The listing builds one solid part. Answer for the finished solid, in the listing's coordinates (mm). Face numbers are marked on the shaded views. Give positions to 0.01 mm unless a question says otherwise; leave off trailing zeros. Put each result on its own line as item: value. Start each with the question number.
1) A cutting plane is placed at A-A (y = 2.5). Give the number of separate pieces and of enclosed holes in the cut face, then the cut area to 3 significant figures.
2) For a pull along Z with two mould halves and no side action, classify the marked faces 1 and 2 as released by +Z, released by -Z, zero draft, split by the parting line, or undercut.
3) Find the intervals of material crossed by line 1 along Z through (x, y) = (6, 2); line 2 along X through (y, z) = (4, 35); line 3 along Z through (x, y) = (-2.5, 3), in increasing order. Write a range as from..to.
4) Flat-ended cylindrical pins translate along their axes: pin 1 Ø2.5 at (y, z) = (2, -35) entering from +X; pin 2 Ø4 at (x, z) = (5.13, 14.1) entering from +Y; pin 3 Ø1 at (y, z) = (3, 9.5) entering from -X. Find the tip coordinate at first contact, or state that the pin passes through.
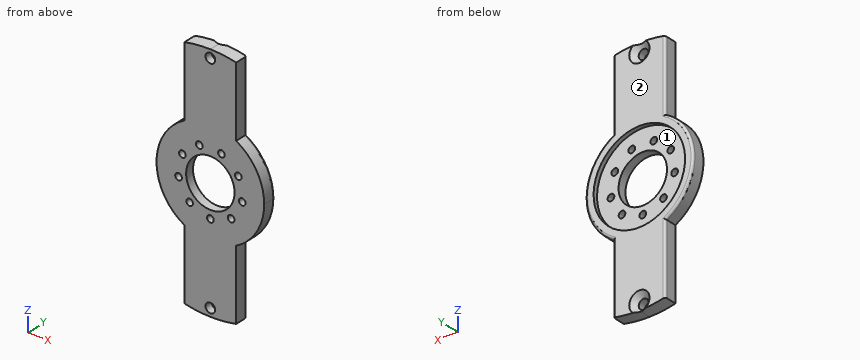
from build123d import *

# Parameters (mm, degrees)
BOSS_EXTRUDE2_DEPTH                             = 6
CSK_FOR_M4_FLAT_HEAD_MACHINE_SCREW1_D           = 4.5
CSK_FOR_M4_FLAT_HEAD_MACHINE_SCREW1_CSINK_D     = 9.4
CSK_FOR_M4_FLAT_HEAD_MACHINE_SCREW1_CSINK_ANGLE = 90
SKETCH7_R                                       = 21.25
CUT_EXTRUDE2_DEPTH                              = 2
SKETCH8_R                                       = 11.25
CUT_EXTRUDE3_DEPTH                              = 62.457302349
SKETCH9_R                                       = 1.55
CUT_EXTRUDE4_DEPTH                              = 62.457302349
FILLET1_R                                       = 1


with BuildPart() as part:
    # Sketch2 → Boss-Extrude2 (new body)
    with BuildSketch(Plane(origin=(0, 0, 0), x_dir=(1, 0, 0), z_dir=(0, 1, 0))):
        with BuildLine():
            ThreePointArc((0, -50), (-6.044327096, -49.633316532), (-12, -48.538644398))
            Line((-12, -48.538644398), (-12, -54.699177325))
            ThreePointArc((-12, -54.699177325), (-6.035149949, -55.673844533), (0, -56))
            Line((0, -56), (0, -54.269322199))
            ThreePointArc((0, -54.269322199), (-2, -52.269322199), (0, -50.269322199))
            Line((0, -50.269322199), (0, -50))
        make_face()
        with BuildLine():
            ThreePointArc((2, -52.269322199), (1.414213562, -50.855108637), (0, -50.269322199))
            Line((0, -50.269322199), (0, -54.269322199))
            ThreePointArc((0, -54.269322199), (1.414213562, -53.683535761), (2, -52.269322199))
        make_face()
        with BuildLine():
            Line((0, -54.269322199), (0, -50.269322199))
            ThreePointArc((0, -50.269322199), (-2, -52.269322199), (0, -54.269322199))
        make_face()
        with BuildLine():
            ThreePointArc((2, -52.269322199), (1.414213562, -50.855108637), (0, -50.269322199))
            Line((0, -50.269322199), (0, -54.269322199))
            ThreePointArc((0, -54.269322199), (1.414213562, -53.683535761), (2, -52.269322199))
        make_face()
        with BuildLine():
            Line((0, -54.269322199), (0, -50.269322199))
            ThreePointArc((0, -50.269322199), (-2, -52.269322199), (0, -54.269322199))
        make_face()
        with BuildLine():
            Line((12, -54.699177325), (12, -48.538644398))
            ThreePointArc((12, -48.538644398), (6.044327096, -49.633316532), (0, -50))
            Line((0, -50), (0, -50.269322199))
            ThreePointArc((0, -50.269322199), (1.414213562, -50.855108637), (2, -52.269322199))
            ThreePointArc((2, -52.269322199), (1.414213562, -53.683535761), (0, -54.269322199))
            Line((0, -54.269322199), (0, -56))
            ThreePointArc((0, -56), (6.035149949, -55.673844533), (12, -54.699177325))
        make_face()
        with BuildLine():
            Line((0, -48.538644398), (-12, -48.538644398))
            ThreePointArc((-12, -48.538644398), (-6.044327096, -49.633316532), (0, -50))
            Line((0, -50), (0, -48.538644398))
        make_face()
        with BuildLine():
            Line((12, -48.538644398), (0, -48.538644398))
            Line((0, -48.538644398), (0, -50))
            ThreePointArc((0, -50), (6.044327096, -49.633316532), (12, -48.538644398))
        make_face()
        with BuildLine():
            ThreePointArc((0, -25), (-6.193028137, -24.220784514), (-12, -21.931712199))
            Line((-12, -21.931712199), (-12, -48.538644398))
            Line((-12, -48.538644398), (0, -48.538644398))
            Line((0, -48.538644398), (0, -25))
        make_face()
        with BuildLine():
            ThreePointArc((12, -21.931712199), (6.193028137, -24.220784514), (0, -25))
            Line((0, -25), (0, -48.538644398))
            Line((0, -48.538644398), (12, -48.538644398))
            Line((12, -48.538644398), (12, -21.931712199))
        make_face()
        with BuildLine():
            Line((0, -48.538644398), (-12, -48.538644398))
            ThreePointArc((-12, -48.538644398), (-6.044327096, -49.633316532), (0, -50))
            Line((0, -50), (0, -48.538644398))
        make_face()
        with BuildLine():
            Line((12, -48.538644398), (0, -48.538644398))
            Line((0, -48.538644398), (0, -50))
            ThreePointArc((0, -50), (6.044327096, -49.633316532), (12, -48.538644398))
        make_face()
        with BuildLine():
            ThreePointArc((-12, 48.538644398), (-6.044327096, 49.633316532), (0, 50))
            Line((0, 50), (0, 50.269322199))
            ThreePointArc((0, 50.269322199), (-2, 52.269322199), (0, 54.269322199))
            Line((0, 54.269322199), (0, 56))
            ThreePointArc((0, 56), (-6.035149949, 55.673844533), (-12, 54.699177325))
            Line((-12, 54.699177325), (-12, 48.538644398))
        make_face()
        with BuildLine():
            ThreePointArc((0, 54.269322199), (-2, 52.269322199), (0, 50.269322199))
            Line((0, 50.269322199), (0, 54.269322199))
        make_face()
        with BuildLine():
            Line((0, 54.269322199), (0, 50.269322199))
            ThreePointArc((0, 50.269322199), (1.414213562, 50.855108637), (2, 52.269322199))
            ThreePointArc((2, 52.269322199), (1.414213562, 53.683535761), (0, 54.269322199))
        make_face()
        with BuildLine():
            ThreePointArc((0, 54.269322199), (-2, 52.269322199), (0, 50.269322199))
            Line((0, 50.269322199), (0, 54.269322199))
        make_face()
        with BuildLine():
            Line((0, 54.269322199), (0, 50.269322199))
            ThreePointArc((0, 50.269322199), (1.414213562, 50.855108637), (2, 52.269322199))
            ThreePointArc((2, 52.269322199), (1.414213562, 53.683535761), (0, 54.269322199))
        make_face()
        with BuildLine():
            Line((0, 50.269322199), (0, 50))
            ThreePointArc((0, 50), (6.044327096, 49.633316532), (12, 48.538644398))
            Line((12, 48.538644398), (12, 54.699177325))
            ThreePointArc((12, 54.699177325), (6.035149949, 55.673844533), (0, 56))
            Line((0, 56), (0, 54.269322199))
            ThreePointArc((0, 54.269322199), (1.414213562, 53.683535761), (2, 52.269322199))
            ThreePointArc((2, 52.269322199), (1.414213562, 50.855108637), (0, 50.269322199))
        make_face()
        with BuildLine():
            Line((-12, 48.538644398), (0, 48.538644398))
            Line((0, 48.538644398), (0, 50))
            ThreePointArc((0, 50), (-6.044327096, 49.633316532), (-12, 48.538644398))
        make_face()
        with BuildLine():
            Line((0, 50), (0, 48.538644398))
            Line((0, 48.538644398), (12, 48.538644398))
            ThreePointArc((12, 48.538644398), (6.044327096, 49.633316532), (0, 50))
        make_face()
        with BuildLine():
            Line((-12, 48.538644398), (0, 48.538644398))
            Line((0, 48.538644398), (0, 50))
            ThreePointArc((0, 50), (-6.044327096, 49.633316532), (-12, 48.538644398))
        make_face()
        with BuildLine():
            Line((0, 50), (0, 48.538644398))
            Line((0, 48.538644398), (12, 48.538644398))
            ThreePointArc((12, 48.538644398), (6.044327096, 49.633316532), (0, 50))
        make_face()
        with BuildLine():
            Line((0, 25), (0, 48.538644398))
            Line((0, 48.538644398), (-12, 48.538644398))
            Line((-12, 48.538644398), (-12, 21.931712199))
            ThreePointArc((-12, 21.931712199), (-6.193028137, 24.220784514), (0, 25))
        make_face()
        with BuildLine():
            Line((12, 48.538644398), (0, 48.538644398))
            Line((0, 48.538644398), (0, 25))
            ThreePointArc((0, 25), (6.193028137, 24.220784514), (12, 21.931712199))
            Line((12, 21.931712199), (12, 48.538644398))
        make_face()
        with BuildLine():
            ThreePointArc((12, 21.931712199), (6.193028137, 24.220784514), (0, 25))
            Line((0, 25), (0, 21.25))
            ThreePointArc((0, 21.25), (15.0260191, 15.0260191), (21.25, 0))
            ThreePointArc((21.25, 0), (15.0260191, -15.0260191), (0, -21.25))
            Line((0, -21.25), (0, -25))
            ThreePointArc((0, -25), (6.193028137, -24.220784514), (12, -21.931712199))
            ThreePointArc((12, -21.931712199), (21.505813168, -12.747548784), (25, 0))
            ThreePointArc((25, 0), (21.505813168, 12.747548784), (12, 21.931712199))
        make_face()
        with BuildLine():
            Line((0, 21.25), (0, 25))
            ThreePointArc((0, 25), (-6.193028137, 24.220784514), (-12, 21.931712199))
            ThreePointArc((-12, 21.931712199), (-25, 0), (-12, -21.931712199))
            ThreePointArc((-12, -21.931712199), (-6.193028137, -24.220784514), (0, -25))
            Line((0, -25), (0, -21.25))
            ThreePointArc((0, -21.25), (-21.25, 0), (0, 21.25))
        make_face()
        with BuildLine():
            ThreePointArc((21.25, 0), (15.0260191, 15.0260191), (0, 21.25))
            Line((0, 21.25), (0, 0))
            Line((0, 0), (0, -21.25))
            ThreePointArc((0, -21.25), (15.0260191, -15.0260191), (21.25, 0))
        make_face()
        with BuildLine():
            Line((0, 0), (0, 21.25))
            ThreePointArc((0, 21.25), (-21.25, 0), (0, -21.25))
            Line((0, -21.25), (0, 0))
        make_face()
        with BuildLine():
            ThreePointArc((21.25, 0), (15.0260191, 15.0260191), (0, 21.25))
            Line((0, 21.25), (0, 0))
            Line((0, 0), (0, -21.25))
            ThreePointArc((0, -21.25), (15.0260191, -15.0260191), (21.25, 0))
        make_face()
        with BuildLine():
            Line((0, 0), (0, 21.25))
            ThreePointArc((0, 21.25), (-21.25, 0), (0, -21.25))
            Line((0, -21.25), (0, 0))
        make_face()
        with BuildLine():
            ThreePointArc((12, 21.931712199), (6.193028137, 24.220784514), (0, 25))
            Line((0, 25), (0, 21.25))
            ThreePointArc((0, 21.25), (15.0260191, 15.0260191), (21.25, 0))
            ThreePointArc((21.25, 0), (15.0260191, -15.0260191), (0, -21.25))
            Line((0, -21.25), (0, -25))
            ThreePointArc((0, -25), (6.193028137, -24.220784514), (12, -21.931712199))
            ThreePointArc((12, -21.931712199), (21.505813168, -12.747548784), (25, 0))
            ThreePointArc((25, 0), (21.505813168, 12.747548784), (12, 21.931712199))
        make_face()
        with BuildLine():
            Line((0, 21.25), (0, 25))
            ThreePointArc((0, 25), (-6.193028137, 24.220784514), (-12, 21.931712199))
            ThreePointArc((-12, 21.931712199), (-25, 0), (-12, -21.931712199))
            ThreePointArc((-12, -21.931712199), (-6.193028137, -24.220784514), (0, -25))
            Line((0, -25), (0, -21.25))
            ThreePointArc((0, -21.25), (-21.25, 0), (0, 21.25))
        make_face()
    extrude(amount=BOSS_EXTRUDE2_DEPTH)

    # CSK for M4 Flat Head Machine Screw1 (through all)
    with Locations(Plane(origin=(0, 6, 0), x_dir=(1, 0, 0), z_dir=(0, 1, 0))):
        with Locations((0, 52.269322197)):
            csk_for_m4_flat_head_machine_screw1 = CounterSinkHole(CSK_FOR_M4_FLAT_HEAD_MACHINE_SCREW1_D / 2, CSK_FOR_M4_FLAT_HEAD_MACHINE_SCREW1_CSINK_D / 2, counter_sink_angle=CSK_FOR_M4_FLAT_HEAD_MACHINE_SCREW1_CSINK_ANGLE)

    # Mirror1: CSK for M4 Flat Head Machine Screw1 across plane
    add(csk_for_m4_flat_head_machine_screw1.mirror(Plane.XY), mode=Mode.SUBTRACT)

    # Sketch7 → Cut-Extrude2 (cut)
    with BuildSketch(Plane(origin=(0, 6, 0), x_dir=(1, 0, 0), z_dir=(0, 1, 0))):
        with Locations(Location((0, 0, 0), (0, 0, 270))):
            Circle(SKETCH7_R)
    extrude(amount=-CUT_EXTRUDE2_DEPTH, mode=Mode.SUBTRACT)

    # Sketch8 → Cut-Extrude3 (cut, through all)
    with BuildSketch(Plane(origin=(0, 4, 0), x_dir=(1, 0, 0), z_dir=(0, 1, 0))):
        with Locations(Location((0, 0, 0), (0, 0, 270))):
            Circle(SKETCH8_R)
    extrude(amount=-CUT_EXTRUDE3_DEPTH, mode=Mode.SUBTRACT)

    # Sketch9 → Cut-Extrude4 (cut, through all)
    with BuildSketch(Plane(origin=(0, 4, 0), x_dir=(1, 0, 0), z_dir=(0, 1, 0))):
        with Locations(Location((0, 15, 0), (0, 0, 270))):
            Circle(SKETCH9_R)
        with Locations(Location((9.641814145, 11.490666647, 0), (0, 0, 270))):
            Circle(SKETCH9_R)
        with Locations(Location((14.772116295, 2.604722665, 0), (0, 0, 270))):
            Circle(SKETCH9_R)
        with Locations(Location((12.990381057, -7.5, 0), (0, 0, 270))):
            Circle(SKETCH9_R)
        with Locations(Location((5.13030215, -14.095389312, 0), (0, 0, 270))):
            Circle(SKETCH9_R)
        with Locations(Location((-5.13030215, -14.095389312, 0), (0, 0, 270))):
            Circle(SKETCH9_R)
        with Locations(Location((-12.990381057, -7.5, 0), (0, 0, 270))):
            Circle(SKETCH9_R)
        with Locations(Location((-14.772116295, 2.604722665, 0), (0, 0, 270))):
            Circle(SKETCH9_R)
        with Locations(Location((-9.641814145, 11.490666647, 0), (0, 0, 270))):
            Circle(SKETCH9_R)
    extrude(amount=-CUT_EXTRUDE4_DEPTH, mode=Mode.SUBTRACT)

    # Fillet1
    fillet1_edges = [part.edges().sort_by_distance(p)[0] for p in [
        (-12, 6, -38.315444762),
        (-25, 6, 0),
        (-12, 6, 38.315444762),
        (12, 6, 38.315444762),
        (25, 6, 0),
        (12, 6, -38.315444762),
    ]]
    fillet(fillet1_edges, radius=FILLET1_R)


solid = part.part
Reply:
1. separate pieces: 1
1. enclosed holes: 12
1. area: 2,980 mm2
2. face 1: undercut
2. face 2: zero draft
3. line 1: z = -55.68..-9.52, 9.52..12.81, 15.38..55.68
3. line 2: x = -12..12
3. line 3: z = -55.94..-10.97, 10.97..55.94
4. pin 1: stops at x = 12
4. pin 2: stops at y = 4
4. pin 3: stops at x = -23.32
